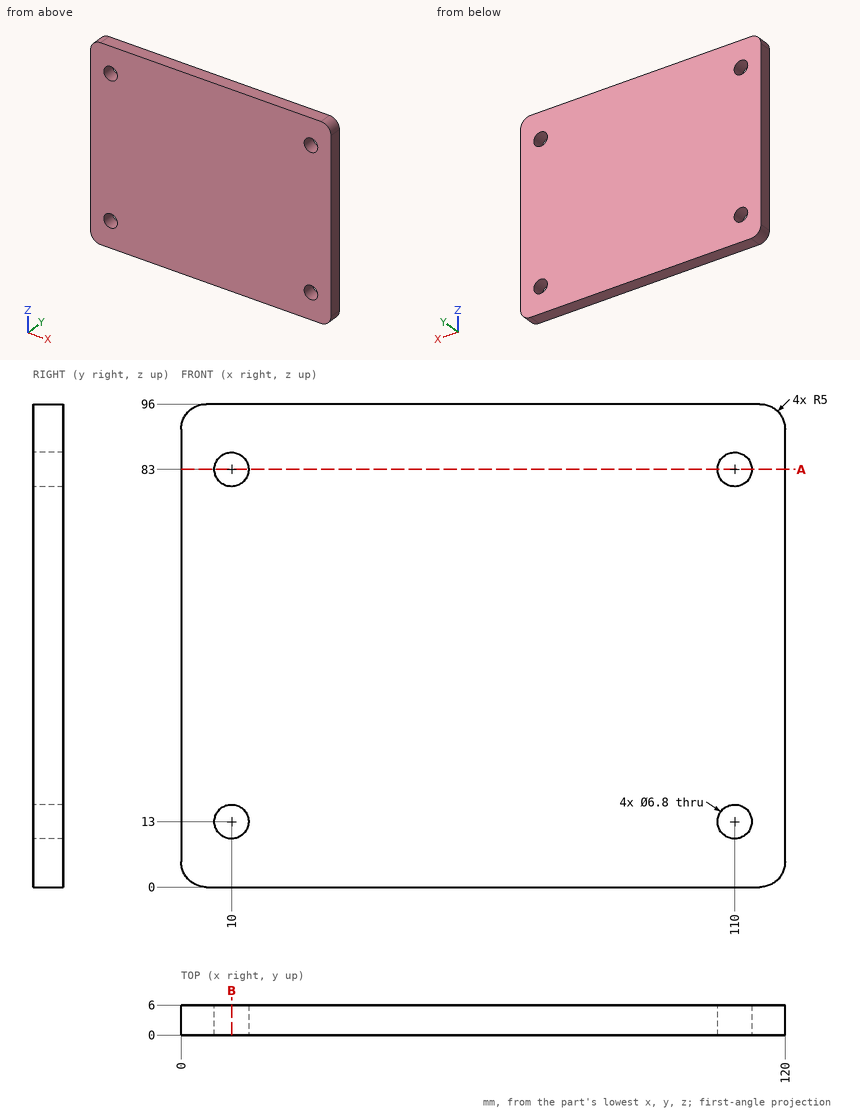
Design review of the part shown in the three views and the two pictorial views. Dimensions are in mm from the part's minimum x, y and z. Round coordinates to 2 decimals unless told otherwise and drop trailing zeros. Loops run counter-clockwise (first coordinate to the right, second up) from the corner with the lowest first, then second, coordinate; pieces in that order, holes last. Notation, with made-up numbers: (72, 1) - (80, 1) arc R14 cw to (80, 19) - close; hole circle Ø1 at (62, 20.5). An arc over 180 degrees is marked (long way). Use one line per item in the form item = value.
1) Clearance check with a flat-ended pin moving along its axis: P1, Ø5.5, axis at x = 110, z = 83, coming from the +Y side. State where the tip first meets the part, or that it passes through.
Solutions:
P1 = through
2) We need section B-B on x = 10. Write out the cut boundary in (y, z), then the cut area to 3 significant figures.
Solutions:
outline = (0, 0) - (6, 0) - (6, 9.6) - (0, 9.6) - close; (0, 16.4) - (6, 16.4) - (6, 79.6) - (0, 79.6) - close; (0, 86.4) - (6, 86.4) - (6, 96) - (0, 96) - close
area = 494 mm2
3) We need section A-A on z = 83. Write out the cut boundary in (x, y).
Solutions:
outline = (0, 0) - (6.6, 0) - (6.6, 6) - (0, 6) - close; (13.4, 0) - (106.6, 0) - (106.6, 6) - (13.4, 6) - close; (113.4, 0) - (120, 0) - (120, 6) - (113.4, 6) - close
4) Wall thickness on probe 1 along Z at (x, y) = (10, 4.55); probe 2 along Z at (x, y) = (11, 1.2); probe 3 along X at (y, z) = (1.5, 4): over which ranges is each line inside the solid? List them lowest first.
Solutions:
probe_1 = 0 to 9.6, 16.4 to 79.6, 86.4 to 96
probe_2 = 0 to 9.75, 16.25 to 79.75, 86.25 to 96
probe_3 = 0.1 to 119.9
